Input: part model. Units: mm. Frame: model coordinates. Face numbers are marked on the shaded views. A direction names the side the tool comes from. Round coordinates to 2 decimals unless told otherwise and drop trailing zeros. Write each loop counter-clockwise with the first axis right and the second up, starting at its lowest first coordinate (ties: lowest second). Pieces come first, ordered by that corner, then holes. Notation, with made-up numbers: (-27.75, -28) -> (-10.75, -28) arc R36 ccw to (-10.75, 8) -> close; hole circle Ø2 at (74.25, 55). An arc over 180 degrees is marked (long way). Use CSV: the item, a comma, the result in double quotes.
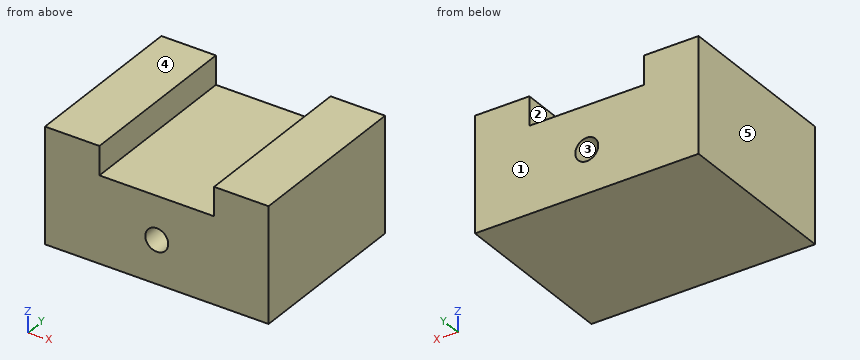
```python
from build123d import *

# Parameters (mm, degrees)
SKETCH_1_W          = 78
SKETCH_1_H          = 60
EXTRUDE_1_DEPTH     = 30
SKETCH_2_W          = 19
SKETCH_2_H          = 60
EXTRUDE_2_DEPTH     = 10
SKETCH_3_R          = 4
CUT_EXTRUDE_1_DEPTH = 60


with BuildPart() as part:
    # 草图1 → 凸台-拉伸1 (new body)
    with BuildSketch(Plane.XY):
        Rectangle(SKETCH_1_W, SKETCH_1_H)
    extrude(amount=EXTRUDE_1_DEPTH)

    # 草图2 → 凸台-拉伸2 (add)
    with BuildSketch(Plane.XY.offset(30)):
        with Locations((29.5, 0)):
            Rectangle(SKETCH_2_W, SKETCH_2_H)
        with Locations((-29.5, 0)):
            Rectangle(SKETCH_2_W, SKETCH_2_H)
    extrude(amount=EXTRUDE_2_DEPTH)

    # 草图3 → 切除-拉伸1 (cut)
    with BuildSketch(Plane(origin=(0, 30, 0), x_dir=(1, 0, 0), z_dir=(0, 1, 0))):
        with Locations(Location((0, -15, 0), (0, 0, 270))):
            Circle(SKETCH_3_R)
    extrude(amount=-CUT_EXTRUDE_1_DEPTH, mode=Mode.SUBTRACT)


solid = part.part
```
Item 1: Section query A-A on x = 0. Return the cut outline in (y, z).
Worked answers:
outline,"(-30, 0) -> (30, 0) -> (30, 11) -> (-30, 11) -> close; (-30, 19) -> (30, 19) -> (30, 30) -> (-30, 30) -> close"
Item 2: Line query: line 1 (X direction, y = -16, z = 15); line 2 (X direction, y = 2, z = 35.5); line 3 (Z direction, x = -4.5, y = 19.5). Output: solid intervals per line, ascending.
Worked answers:
line 1,"x = -39 to -4, 4 to 39"
line 2,"x = -39 to -20, 20 to 39"
line 3,"z = 0 to 30"
Item 3: Section query C-C on y = -18. Return the cut outline in (x, z).
Worked answers:
outline,"(-39, 0) -> (39, 0) -> (39, 40) -> (20, 40) -> (20, 30) -> (-20, 30) -> (-20, 40) -> (-39, 40) -> close; hole circle Ø8 at (0, 15)"
Item 4: Section query B-B on z = 36. Return the cut outline in (x, y).
Worked answers:
outline,"(-39, -30) -> (-20, -30) -> (-20, 30) -> (-39, 30) -> close; (20, -30) -> (39, -30) -> (39, 30) -> (20, 30) -> close"
Item 5: Set-up query: the marked faces 1 and 2. Return all of +Z, -Z, +X, -X, +Y, -Y with unobstructed straight access to the full face (end or side cutting, diameter ignored); none if empty.
Worked answers:
face 1,"+Z, -Z, +X, -X, +Y"
face 2,"+Z, +Y, -Y"
Item 6: Section query D-D on x = -13. Return the cut outline in (y, z), plus the area to 3 significant figures.
Worked answers:
outline,"(-30, 0) -> (30, 0) -> (30, 30) -> (-30, 30) -> close"
area,"1,800 mm²"
Item 7: Pull-direction query (X, two-part tool) for the marked faces 3, 4 and 5; classes: +X half, -X half, draft (parallel to the pull), parting line (faces both ways), or undercut.
Worked answers:
face 3,"undercut"
face 4,"draft"
face 5,"-X half"
Item 8: First-contact query: pin 1 Ø12 at (x, y) = (4.5, -12.5) entering from +Z. Flat tip, straight axial feed; report the tip coordinate or a pass-through.
Worked answers:
pin 1,"stops at z = 30"
